```python
from build123d import *

# Parameters (mm, degrees)
SKETCH1_W           = 50
SKETCH1_H           = 50
BOSS_EXTRUDE1_DEPTH = 150
SKETCH2_R           = 15
CUT_EXTRUDE1_DEPTH  = 100


with BuildPart() as part:
    # Sketch1 → Boss-Extrude1 (new body)
    with BuildSketch(Plane(origin=(0, 0, 0), x_dir=(1, 0, 0), z_dir=(0, 1, 0))):
        with Locations((-27.798692914, 7.251418332)):
            Rectangle(SKETCH1_W, SKETCH1_H)
    extrude(amount=BOSS_EXTRUDE1_DEPTH)

    # Sketch2 → Cut-Extrude1 (cut)
    with BuildSketch(Plane.XZ):
        with Locations((-27.798692914, -7.251418332)):
            Circle(SKETCH2_R)
    extrude(amount=-CUT_EXTRUDE1_DEPTH, mode=Mode.SUBTRACT)


solid = part.part
```
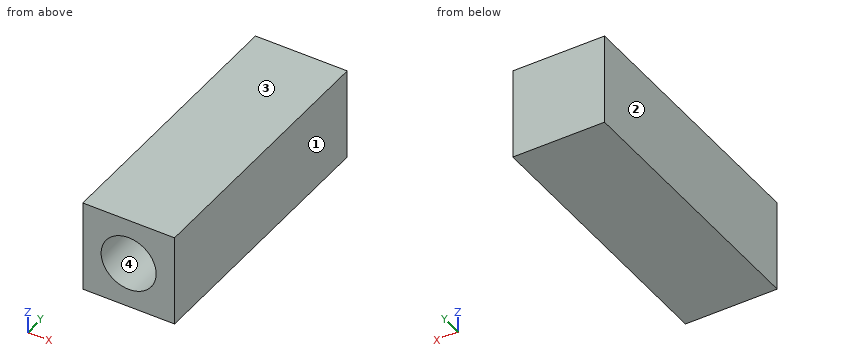
Geometry check sheet. Reference: the model listing, model coordinates, mm. Face numbers are marked on the shaded views. Give positions to 0.01 mm unless a question says otherwise; leave off trailing zeros. Order: outer loops, then holes, each group sorted by start corner. A loop starts at its lowest first (then second) coordinate and runs counter-clockwise, first axis right, second up. Notation, with made-up numbers: (17, -12) - (28, -12) arc R21 ccw to (28, 2) - close; hole circle Ø4 at (-25, 10). An arc over 180 degrees is marked (long way). Write item = value, one per line. Start each with the question number.
1) Draft check along X on the marked faces 1, 2, 3 and 4. Enter one of: released by +X, released by -X, zero draft, split by the parting line, or undercut.
2) Scan lines: L1, parallel to Z at x = -24, y = 53; L2, parallel to X at y = 93.5, z = 2; L3, parallel to Z at x = -38, y = 57. Record each from-to range of solid material in increasing order.
3) Section check C-C (y = 50). Enter the section's corners in (x, z).
4) Section check B-B (z = -3.5). Enter the section's corners in (x, y), then the cut area to 3 significant figures.
5) Section check A-A (x = -26). Enter the section's corners in (y, z), then the cut area to 3 significant figures.
Geometry check:
q1.face_1 = released by +X
q1.face_2 = released by -X
q1.face_3 = zero draft
q1.face_4 = undercut
q2.L1 = -32.25 to -21.76, 7.26 to 17.75
q2.L2 = -52.8 to -39.61, -15.99 to -2.8
q2.L3 = -32.25 to -18.25, 3.75 to 17.75
q3.outline = (-52.8, -32.25) - (-2.8, -32.25) - (-2.8, 17.75) - (-52.8, 17.75) - close; hole circle Ø30 at (-27.8, -7.25)
q4.outline = (-52.8, 0) - (-42.32, 0) - (-42.32, 100) - (-13.28, 100) - (-13.28, 0) - (-2.8, 0) - (-2.8, 150) - (-52.8, 150) - close
q4.area = 4,600 mm2
q5.outline = (0, -32.25) - (150, -32.25) - (150, 17.75) - (0, 17.75) - (0, 7.64) - (100, 7.64) - (100, -22.14) - (0, -22.14) - close
q5.area = 4,520 mm2
